Autodesk Inventor part; units mm, degrees
ref_plane "YZ Plane" through (0, 0, 0) normal (1, 0, 0) x (0, 1, 0)
ref_plane "XZ Plane" through (0, 0, 0) normal (0, 1, 0) x (-1, 0, 0)
ref_plane "XY Plane" through (0, 0, 0) normal (0, 0, 1) x (1, 0, 0)
sketch "Sketch1" plane through (0, 0, 0) normal (0, 0, 1) x (1, 0, 0)
  line L0 (0, 251.46) -> (0, -264.16)
  line L1 (-361.3785, 0) -> (361.3785, 0)
  line L2 (177.8, -190.5) -> (-177.8, -190.5)
  line L3 (-177.8, -190.5) -> (-177.8, 177.8)
  line L4 (-177.8, 177.8) -> (177.8, 177.8)
  line L5 (177.8, 177.8) -> (177.8, -190.5)
  line L6 (143.51, -143.511) -> (-143.51, -143.511) construction
  line L7 (-143.51, -143.511) -> (-143.51, 143.509) construction
  line L8 (-143.51, 143.509) -> (143.51, 143.509) construction
  line L9 (143.51, 143.509) -> (143.51, -143.511) construction
  line L10 (-177.8, 177.8) -> (-177.8, 177.8)
  line L11 (-177.8, -190.5) -> (-177.8, 177.8)
  line L12 (177.8, 177.8) -> (177.8, 177.8)
  line L13 (177.8, -190.5) -> (177.8, 177.8)
  line L14 (-165.1, -158.75) -> (165.1, -158.75) construction
  line L15 (165.1, -158.75) -> (165.1, 158.75) construction
  line L16 (165.1, 158.75) -> (-165.1, 158.75) construction
  line L17 (-165.1, 158.75) -> (-165.1, -158.75) construction
  line L18 (144.4625, 143.509) -> (-144.4625, 143.509)
  line L19 (-144.4625, 143.509) -> (-144.4625, -190.5)
  line L20 (-144.4625, -190.5) -> (144.4625, -190.5)
  line L21 (144.4625, -190.5) -> (144.4625, 143.509)
  line L22 (144.4625, 143.509) -> (-144.4625, -190.5) construction
  line L23 (-144.4625, 143.509) -> (144.4625, -190.5) construction
  circle A0 centre (-209.55, 0) radius 48.5775
  circle A1 centre (209.55, 0) radius 48.5775
  line L24 (-65.455, 153.009) -> (-55.955, 153.009) construction
  line L25 (0, 177.8) -> (0, 143.509)
  point P0 (0, 0)
  point P1 (0, -23.4955)
  point P2 (-71.755, 153.009)
  point P3 (-139.7, 158.75)
  point P4 (139.7, 158.75)
  point P5 (0, 158.75)
  point P6 (-88.9, 158.75)
  point P7 (88.9, 158.75)
  point P8 (-165.1, -95.25)
  point P9 (165.1, -95.25)
  dimension "d2" = 355.6
  dimension "d66" = 177.8
  dimension "d70" = 368.3
  dimension "d71" = 177.8
  dimension "d85" = 287.02
  dimension "d86" = 330.2
  dimension "d94" = 288.925
  dimension "d95" = 0
  dimension "d107" = 209.55
  dimension "d108" = 97.155
  dimension "d111" = 209.55
  dimension "d112" = 9.5
  dimension "d113" = 9.5
  dimension "d115" = 15.8
  dimension "d116" = 71.755
  dimension "d124" = 139.7
  dimension "d125" = 139.7
  dimension "d133" = 317.5
  dimension "d134" = 165.1
  dimension "d135" = 158.75
  dimension "d136" = 50.8
  dimension "d137" = 50.8
  dimension "d158" = 63.5
  dimension "d159" = 63.5
  dimension "d160" = 55.955
extrude "Extrusion1" add sketch "Sketch1" against normal blind 6.35 contours L4 L5 A1 L1 L21 L18 L0 | L0 L18 L19 L1 A0 L3 L4 | L18 L21 L1 L0 | L0 L1 L19 L18 | L1 L21 L2 L0 | L0 L2 L19 L1 | A0 L1 L3 | L5 L1 A1 | L19 L2 L3 A0 L1 | L1 A1 L5 L2 L21 | L1 A0 L3 | L5 A1 L1 picked at (-175.8618, 22.522) picked at (175.8618, 22.522) picked at (-175.8618, -22.522) picked at (175.8618, -22.522)
hole "Hole5" at (-165.1, 158.75, 0) at (165.1, 158.75, 0) at (165.1, -158.75, 0) at (-165.1, -158.75, 0) at (-165.1, -95.25, 0) at (165.1, -95.25, 0) direction (0, 0, -1) diameter 5.1054 end through all
extrude "Extrusion5" cut sketch "Sketch1" against normal up to next contours L18 L21 L1 L0 | L0 L1 L19 L18 | L1 L21 L2 L0 | L0 L2 L19 L1
chamfer "Chamfer3" distance 15.875 angle 60 1 edges at (-144.4625, -190.5, -3.175) measured on face at (-166.6875, -190.5, -4.2333)
chamfer "Chamfer4" distance 15.875 angle 60 1 edges at (144.4625, -190.5, -3.175) measured on face at (155.575, -190.5, -4.2333)
fillet "Fillet8" radius 12.7 4 edges at (160.3375, -190.5, -3.175) (144.4625, -163.0037, -3.175) (-144.4625, -163.0037, -3.175) (-160.3375, -190.5, -3.175)
fillet "Fillet6" radius 12.7 4 edges at (177.8, -190.5, -3.175) (177.8, 177.8, -3.175) (-177.8, -190.5, -3.175) (-177.8, 177.8, -3.175)
fillet "Fillet7" radius 10.16 2 edges at (144.4625, 143.509, -3.175) (-144.4625, 143.509, -3.175)
extrude "Extrusion6" cut sketch "Sketch1" against normal up to next contours A0 L1 L3 | L3 L1 A0 | A1 L1 L5 | L5 L1 A1 | L3 A0 L1 | L1 A0 L3 | L5 A1 L1 | L1 A1 L5
hole "Hole6" at (-143.51, 143.509, 0) at (-65.455, 153.009, 0) at (-55.955, 153.009, 0) direction (0, 0, -1) diameter 1.524 end through all
mirror "Mirror1" about plane through (0, 0, 0) normal (1, 0, 0) of "Hole6"
hole "Hole7" at (-139.7, 158.75, 0) at (139.7, 158.75, 0) at (-88.9, 158.75, 0) at (88.9, 158.75, 0) direction (0, 0, -1) diameter 4.4958 end through all countersink diameter 9.398 countersink angle 90
sketch "Sketch3" plane through (0, 0, 0) normal (0, 0, 1) x (1, 0, 0)
  line L0 (0, 294.3121) -> (0, -274.6479)
  line L1 (-258.445, 0) -> (306.07, 0)
  line L2 (-79.375, 213.0321) -> (225.425, 213.0321)
  line L3 (225.425, 213.0321) -> (225.425, -193.3679)
  line L4 (225.425, -193.3679) -> (-79.375, -193.3679)
  line L5 (-79.375, -193.3679) -> (-79.375, 213.0321)
  line L6 (-177.8, -36.7656) -> (-177.8, -173.3489)
  line L7 (-144.4625, -159.6007) -> (-144.4625, 133.349)
  point P0 (0, 0)
  point P1 (-153.67, -152.4)
  dimension "d138" = 304.8
  dimension "d139" = 406.4
  dimension "d140" = 79.375
  dimension "d144" = 24.13
  dimension "d145" = 152.4
  dimension "d157" = 9.2075
extrude "Extrusion7" cut sketch "Sketch3" against normal up to next
fillet "Fillet9" radius 3.175 2 edges at (-79.375, 143.509, -3.175) (-79.375, 177.8, -3.175)
hole "Hole8" at (-153.67, -152.4, 0) direction (0, 0, -1) diameter 3.2766 end through all
pattern_linear "Rectangular Pattern3" count 10 spacing 12.7 along (0, 1, 0) of "Hole8"
chamfer "Chamfer5" distance 2.4384 angle 45 2 edges at (-139.7, 160.9979, -6.35) (-88.9, 160.9979, -6.35)
ref_plane "Work Plane1" through (0, 0, 0) normal (1, 0, 0) x (0, 1, 0)
properties material "ACETAL COPOLYMER, WHITE"
Check sheet for the modelled part. Datum: model origin and axes. Units: mm. A direction names the side the tool comes from. Coordinates: 2 decimals unless noted, no trailing zeros. Loops run counter-clockwise (first coordinate to the right, second up) from the corner with the lowest first, then second, coordinate; pieces in that order, holes last. Notation, with made-up numbers: (39, -35) -> (79, -35) arc R13 ccw to (79, -19) -> close; hole circle Ø3 at (14, 67). An arc over 180 degrees is marked (long way). Answer in a Markdown table with one row per item.
1. Material ranges on line 1 along X through (y, z) = (-50.8, -4.5); line 2 along X through (y, z) = (-158.75, -3); line 3 along Y through (x, z) = (-165.1, -5), recorded low to high. Write a range as [from, to].
Check values:
| item | result |
|---|---|
| line 1 | x = [-177.8, -155.31], [-152.03, -144.46] |
| line 2 | x = [-177.8, -167.65], [-162.55, -144.46] |
| line 3 | y = [-186.05, -161.3], [-156.2, -97.8], [-92.7, -19.6], [19.6, 156.2], [161.3, 177.8] |
2. Sectioned sample at A-A, the plane y = -69. Record the boundary of the cut face in (x, z), then the cut area to 3 significant figures.
Check values:
| item | result |
|---|---|
| outline | (-177.8, -6.35) -> (-144.46, -6.35) -> (-144.46, 0) -> (-177.8, 0) -> close |
| area | 212 mm2 |
3. Go/stop test with flat-tipped pins: pin 1 (1.9 mm diameter, centred on y = 36.5, z = -3, fed in from +X); pin 2 (3 mm diameter, centred on x = -105.5, z = -3.5, fed in from -Y); pin 3 (6 mm diameter, centred on x = -88.9, y = 158.75, fed in from +Z). Record where each tip stops, or that it passes through.
Check values:
| item | result |
|---|---|
| pin 1 | stops at x = -144.46 |
| pin 2 | stops at y = 143.51 |
| pin 3 | stops at z = -1.7 |
4. Access from +Z, -Z, +X, -X, +Y, -Y to the whole of each face (thin tool, end or side, straight path). Record for faces 4 (the face through (-90.92, 157.46, -4.06)), 5 (the face through (-108, 143.509, -3)).
Check values:
| item | result |
|---|---|
| face 4 | -Z |
| face 5 | +Z, -Z, +X, -Y |
5. Sectioned sample at B-B, the plane x = -123. Record the boundary of the cut face in (y, z), then the cut area to 3 significant figures.
Check values:
| item | result |
|---|---|
| outline | (143.51, -6.35) -> (177.8, -6.35) -> (177.8, 0) -> (143.51, 0) -> close |
| area | 218 mm2 |
6. Sectioned sample at C-C, the plane z = -5. Give the number of separate pieces and of enclosed holes in the cut face, then the cut area to 3 significant figures.
Check values:
| item | result |
|---|---|
| separate pieces | 1 |
| enclosed holes | 16 |
| area | 13,100 mm2 |
7. Release check for a two-part mould opening along X. For faces 1 (the face through (-141.161, 160.656, -2.298)), 2 (the face through (-177.8, -106, -3)), 3 (the face through (-150.08, -172.73, -3.13)) record: released by +X, released by -X, zero draft, split by the parting line, or undercut.
Check values:
| item | result |
|---|---|
| face 1 | undercut |
| face 2 | released by -X |
| face 3 | released by +X |
